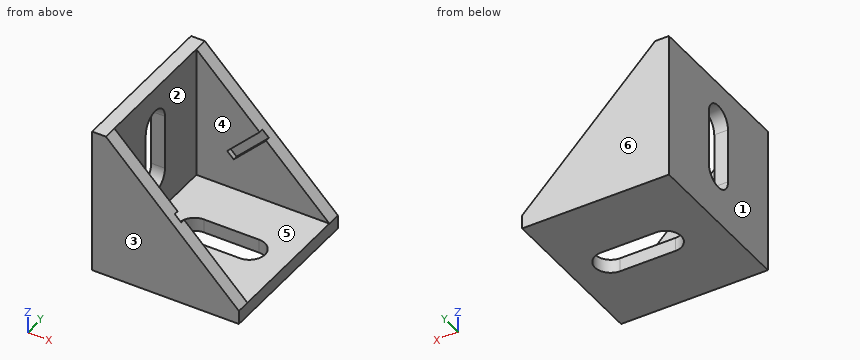
from build123d import *

# Parameters (mm, degrees)
F1_DEPTH  = 35
F2_T      = 3
F4_DEPTH  = 3
F6_DEPTH  = 3
F8_DEPTH  = 1
F10_DEPTH = 1


# Not quite as in the source:
# - a shell that OpenCascade refuses in one call is made with other operations: the cavity is built on its own and cut out


with BuildPart() as f1:
    # F0 (on Front) → F1 (new body)
    with BuildSketch(Plane.XZ):
        Polygon((0, 32), (0, 0), (32, 0), (32, 3), (3, 32), align=None)
    extrude(amount=F1_DEPTH)

    # F2: shell of thickness 3, made by hand


with BuildPart() as f2_core1:
    # F2_t2: copy of F1
    add(f1.part)

    # the walls: a layer under each face that stays
    f2_faces = [f2_core1.faces().sort_by_distance(p)[0] for p in [
        (0, -17.5, 16),
        (16, -17.5, 0),
        (16, 0, 16),
        (16, -35, 16),
    ]]
    thicken(f2_faces, amount=-F2_T, mode=Mode.SUBTRACT)


with BuildPart() as f1_1:
    add(f1.part)

    # what is left inside the walls is the cavity
    f2_cavity = [f2_core1.part.solids().sort_by_distance(p)[0] for p in [
        (17.478787, -22.333333, 17.478787),
    ]]
    add(f2_cavity, mode=Mode.SUBTRACT)

    # F3 (on face) → F4 (cut)
    with BuildSketch(Plane.XY.offset(3)):
        with BuildLine():
            Line((11.5, -20.9), (23.5, -20.9))
            ThreePointArc((23.5, -20.9), (26.9, -17.5), (23.5, -14.1))
            Line((23.5, -14.1), (11.5, -14.1))
            ThreePointArc((11.5, -14.1), (8.1, -17.5), (11.5, -20.9))
        make_face()
    extrude(amount=-F4_DEPTH, mode=Mode.SUBTRACT)

    # F5 (on face) → F6 (cut)
    with BuildSketch(Plane.YZ.offset(3)):
        with BuildLine():
            Line((-14.1, 11.5), (-14.1, 23.5))
            ThreePointArc((-14.1, 23.5), (-17.5, 26.9), (-20.9, 23.5))
            Line((-20.9, 23.5), (-20.9, 11.5))
            ThreePointArc((-20.9, 11.5), (-17.5, 8.1), (-14.1, 11.5))
        make_face()
    extrude(amount=-F6_DEPTH, mode=Mode.SUBTRACT)

    # F7 (on face) → F8 (cut)
    with BuildSketch(Plane.XZ.offset(3)):
        Polygon((11.1360389693, 9.7218254069), (18.2071067812, 16.7928932188), (16.7928932188, 18.2071067812), (9.7218254069, 11.1360389693), align=None)
    extrude(amount=-F8_DEPTH, mode=Mode.SUBTRACT)

    # F9 (on face) → F10 (cut)
    with BuildSketch(Plane(origin=(0, -32, 0), x_dir=(-1, 0, 0), z_dir=(0, 1, 0))):
        Polygon((-16.7928932188, 18.2071067812), (-18.2071067812, 16.7928932188), (-11.1360389693, 9.7218254069), (-9.7218254069, 11.1360389693), align=None)
    extrude(amount=-F10_DEPTH, mode=Mode.SUBTRACT)


solid = f1_1.part
Could you check a few things on this model? Use its own coordinates, in mm. Face numbers are marked on the shaded views. A direction names the side the tool comes from. Give positions to 0.01 mm unless a question says otherwise; leave off trailing zeros. Order: outer loops, then holes, each group sorted by start corner. A loop starts at its lowest first (then second) coordinate and runs counter-clockwise, first axis right, second up. Notation, with made-up numbers: (-15.75, -8.5) -> (-2.75, -8.5) arc R16 ccw to (-2.75, 21.5) -> close; hole circle Ø9 at (76, -1.75). An arc over 180 degrees is marked (long way). Return JSON: item names as keys, results as strings.
1. Imagine slicing it at A-A on y = -17.5. List the corners of the cut face in (x, z) for me.
Answer list:
{"outline": "(0, 0) -> (8.1, 0) -> (8.1, 3) -> (3, 3) -> (3, 8.1) -> (0, 8.1) -> close; (0, 26.9) -> (3, 26.9) -> (3, 32) -> (0, 32) -> close; (26.9, 0) -> (32, 0) -> (32, 3) -> (26.9, 3) -> close"}
2. On a 3-axis mill with a long thin cutter (end or side, diameter ignored), from which of +Z, -Z, +X, -X, +Y, -Y can I reach the whole of each face in a straight line? I mean the marked faces 5 and 6. Say none if no direction works.
Answer list:
{"face 5": "+Z, +X", "face 6": "+Z, -Z, +X, -X, +Y"}
3. Imagine slicing it at D-D on x = 4. List the corners of the cut face in (y, z) for me, then the cut area to 3 significant figures.
Answer list:
{"outline": "(-35, 0) -> (0, 0) -> (0, 31) -> (-3, 31) -> (-3, 3) -> (-32, 3) -> (-32, 31) -> (-35, 31) -> close", "area": "273 mm2"}
4. Imagine slicing it at B-B on x = 26. List the corners of the cut face in (y, z) for me.
Answer list:
{"outline": "(-35, 0) -> (-19.8, 0) -> (-19.8, 3) -> (-32, 3) -> (-32, 9) -> (-35, 9) -> close; (-15.2, 0) -> (0, 0) -> (0, 9) -> (-3, 9) -> (-3, 3) -> (-15.2, 3) -> close"}
5. For pin 1 Ø3 at (x, z) = (4.5, 27.5) entering from +Y; pin 2 Ø12 at (x, y) = (16, -10.5) entering from +Z; pin 3 Ø3 at (y, z) = (-20, 11.5) entering from +X, each with a flat end and sliding along its axis, tell me the tip position at first contact or that it passes through.
Answer list:
{"pin 1": "stops at y = 0", "pin 2": "stops at z = 3", "pin 3": "stops at x = 3"}
6. Thinking about a two-plate mould opening in Y: for the marked faces 1, 2, 3 and 4, which applies, pulls with the +Y half, pulls with the -Y half, needs draft (parallel to the pull), parting line crosses it, or undercut?
Answer list:
{"face 1": "needs draft", "face 2": "undercut", "face 3": "pulls with the -Y half", "face 4": "undercut"}
7. Imagine slicing it at C-C on z = 24. List the corners of the cut face in (x, y) for me, then the cut area to 3 significant figures.
Answer list:
{"outline": "(0, -35) -> (11, -35) -> (11, -32) -> (3, -32) -> (3, -20.86) -> (0, -20.86) -> close; (0, -14.14) -> (3, -14.14) -> (3, -3) -> (11, -3) -> (11, 0) -> (0, 0) -> close", "area": "133 mm2"}
8. I need wall thicknesses on line 1 (Y direction, x = 5.5, z = 17.5); line 2 (X direction, y = -9, z = 13.5). Which ranges of each line are inside material? Lowest first, please. Write a range as from..to.
Answer list:
{"line 1": "y = -35..-32, -3..0", "line 2": "x = 0..3"}
